from build123d import *

# Parameters (mm, degrees)
F1_DEPTH = 15.875
F2_R     = 12.7


# Not quite as in the source:
# - a length typed as a fraction of an inch, garbled in the dataset ("3 / 203.2 mm" for 3/8 in), is restored


with BuildPart() as f1:
    # F0 (on Top) → F1 (new body)
    with BuildSketch(Plane.XY):
        Polygon((201.5417389498, 1143), (0, 0), (50.8, 0), (285.3620821836, 1016), (451.3084056164, 1016), (451.3084056164, 1143), align=None)
    extrude(amount=F1_DEPTH)

    # F2
    f2_edges = [f1.edges().sort_by_distance(p)[0] for p in [
        (201.541739, 1143, 7.9375),
        (285.362082, 1016, 7.9375),
        (0, 0, 7.9375),
        (50.8, 0, 7.9375),
    ]]
    fillet(f2_edges, radius=F2_R)


solid = f1.part
Source: CAD feature listing. Evaluate the final solid. Frame: model axes, mm. Coordinates: 2 decimals unless noted, no trailing zeros. Order: outer loops, then holes, each group sorted by start corner. A loop starts at its lowest first (then second) coordinate and runs counter-clockwise, first axis right, second up. Notation, with made-up numbers: M 27.5,-12.5 L 67.5,-12.5 A26 ccw 67.5,17.5 Z; hole C 64.25,-9 d6. An arc over 180 degrees is marked long. Write each question's results on one line, items separated by ' | '. Start each with the question number.
1. Section A-A, the plane z = 5.5. Return the cut outline in (x, y).
2. Section B-B, the plane x = 310. Return the cut outline in (y, z) (3 decimals).
3. Section C-C, the plane y = 784. Return the cut outline in (x, z) (3 decimals), then the cut area to 3 significant figures.
4. Pin query (flat end, axial travel): pin 1 (1.5 mm diameter, centred on y = 656, z = 7, fed in from +X). Return the tip coordinate at first contact, or that it passes through.
5. Material intervals for L1, parallel to Y at x = 312, z = 5.5; L2, parallel to X at y = 438, z = 3; L3, parallel to X at y = 149, z = 15, sorted ascending.
Solution:
1) outline: M 2.63,14.91 A12.7 ccw 15.14,0 L 40.7,0 A12.7 ccw 53.07,9.84 L 283.09,1006.16 A12.7 cw 295.46,1016 L 451.31,1016 L 451.31,1143 L 212.2,1143 A12.7 ccw 199.69,1132.51 Z
2) outline: M 1016,0 L 1143,0 L 1143,15.875 L 1016,15.875 Z
3) outline: M 138.24,0 L 231.801,0 L 231.801,15.875 L 138.24,15.875 Z | area: 1,490 mm²
4) pin 1: x = 202.42
5) L1: 1016 to 1143 | L2: 77.23 to 151.92 | L3: 26.27 to 85.2
